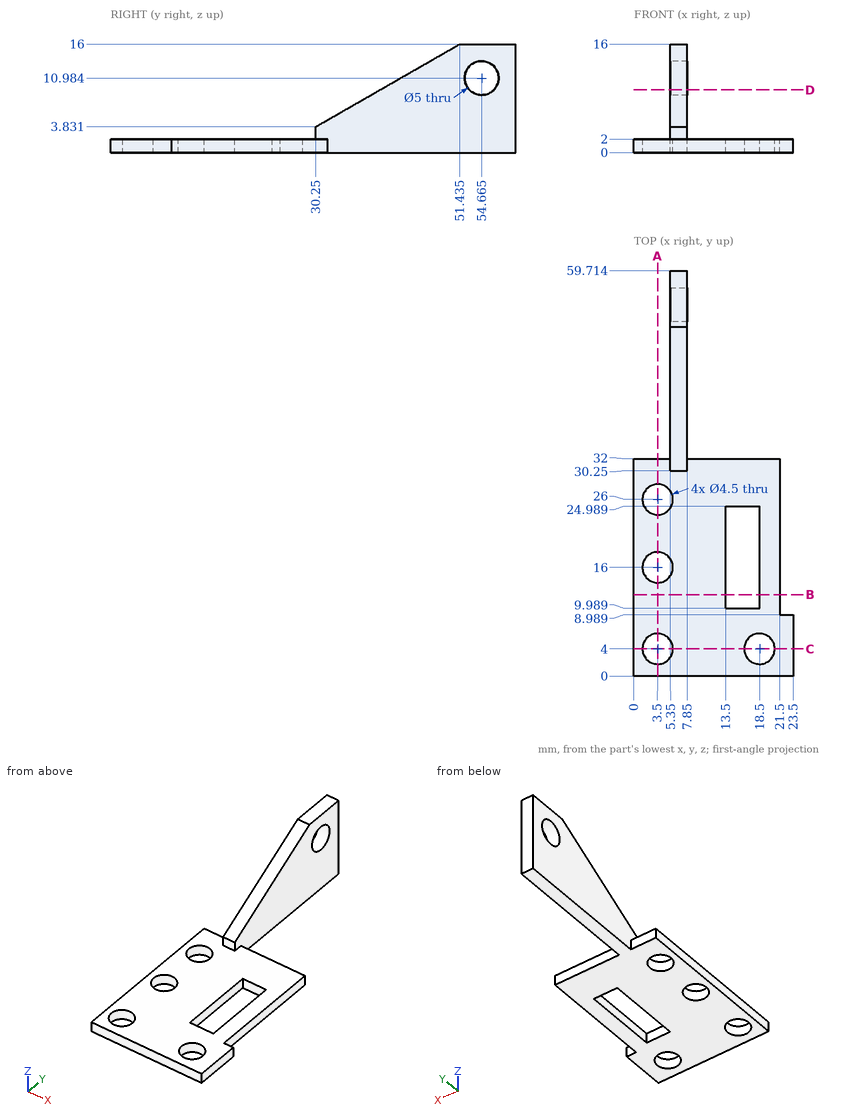
Part print with two shaded views. Sizes in mm from the minimum x, y, z corner. Round coordinates to 2 decimals unless told otherwise and drop trailing zeros. Loops run counter-clockwise (first coordinate to the right, second up) from the corner with the lowest first, then second, coordinate; pieces in that order, holes last.
Item 1: Drill centre lines: line 1 along Y through (x, z) = (3.5, 0.4); line 2 along Y through (x, z) = (2.75, 0.5); line 3 along X through (y, z) = (45, 10.25). Where is each one in solid material? Low to high.
Item 2: Pin check, flat tips, straight feed: P1, Ø1.6, axis at x = 15.5, z = 1, coming from the +Y side; P2, Ø6, axis at y = 54.66, z = 10.98, coming from the +X side; P3, Ø1.6, axis at x = 22.5, z = 0.5, coming from the +Y side. Stop position of each tip, or through.
Item 3: Saw through at B-B (y = 12). List the corners of the cut face in (x, z).
Item 4: Saw through at A-A (x = 3.5). List the corners of the cut face in (y, z), then the cut area to 3 significant figures.
Item 5: Saw through at C-C (y = 4). List the corners of the cut face in (x, z).
Item 6: Saw through at D-D (z = 9.25). List the corners of the cut face in (x, y).
Worked answers:
1. line 1: y = 0 to 1.75, 6.25 to 13.75, 18.25 to 23.75, 28.25 to 32
1. line 2: y = 0 to 1.88, 6.12 to 13.88, 18.12 to 23.88, 28.12 to 32
1. line 3: x = 5.35 to 7.85
2. P1: stops at y = 32
2. P2: stops at x = 7.85
2. P3: stops at y = 8.99
3. outline: (0, 0) - (13.5, 0) - (13.5, 2) - (0, 2) - close; (18.5, 0) - (21.5, 0) - (21.5, 2) - (18.5, 2) - close
4. outline: (0, 0) - (1.75, 0) - (1.75, 2) - (0, 2) - close; (6.25, 0) - (13.75, 0) - (13.75, 2) - (6.25, 2) - close; (18.25, 0) - (23.75, 0) - (23.75, 2) - (18.25, 2) - close; (28.25, 0) - (32, 0) - (32, 2) - (28.25, 2) - close
4. area: 37.0 mm2
5. outline: (0, 0) - (1.25, 0) - (1.25, 2) - (0, 2) - close; (5.75, 0) - (16.25, 0) - (16.25, 2) - (5.75, 2) - close; (20.75, 0) - (23.5, 0) - (23.5, 2) - (20.75, 2) - close
6. outline: (5.35, 39.68) - (7.85, 39.68) - (7.85, 52.86) - (5.35, 52.86) - close; (5.35, 56.47) - (7.85, 56.47) - (7.85, 59.71) - (5.35, 59.71) - close
